```python
from build123d import *

# Parameters (mm, degrees)
F0_R     = 10.3251
F1_DEPTH = 7.9375
F2_W     = 63.5
F2_H     = 7.9375
F3_DEPTH = 68.2625
F4_R     = 9.92251
F5_DEPTH = 88.901
F7_DEPTH = 139.701
F8_DEPTH = 63.5


with BuildPart() as f1:
    # F0 (on Top) → F1 (new body)
    with BuildSketch(Plane.XY):
        with BuildLine():
            Line((63.5, 44.45), (0, 44.45))
            Line((0, 44.45), (0, -44.45))
            Line((0, -44.45), (63.5, -44.45))
            Line((63.5, -44.45), (63.5, -28.575))
            ThreePointArc((63.5, -28.575), (65.359872, -24.084872), (69.85, -22.225))
            Line((69.85, -22.225), (117.475, -22.225))
            ThreePointArc((117.475, -22.225), (139.7, 0), (117.475, 22.225))
            Line((117.475, 22.225), (69.85, 22.225))
            ThreePointArc((69.85, 22.225), (65.359872, 24.084872), (63.5, 28.575))
            Line((63.5, 28.575), (63.5, 44.45))
        make_face()
        with Locations((79.375, 0)):
            Circle(F0_R, mode=Mode.SUBTRACT)
        with Locations((117.475, 0)):
            Circle(F0_R, mode=Mode.SUBTRACT)
    extrude(amount=F1_DEPTH)

    # F2 (on face) → F3 (join)
    with BuildSketch(Plane.XY.offset(7.9375)):
        with Locations((31.75, -40.48125)):
            Rectangle(F2_W, F2_H)
        with Locations((31.75, 40.48125)):
            Rectangle(F2_W, F2_H)
    extrude(amount=F3_DEPTH)

    # F4 (on face) → F5 (cut, through all)
    with BuildSketch(Plane.XZ.offset(44.45)):
        with BuildLine():
            ThreePointArc((0, 44.45), (9.29936, 66.90064), (31.75, 76.2))
            Line((31.75, 76.2), (0, 76.2))
            Line((0, 76.2), (0, 44.45))
        make_face()
        with BuildLine():
            ThreePointArc((31.75, 76.2), (54.20064, 66.90064), (63.5, 44.45))
            Line((63.5, 44.45), (63.5, 76.2))
            Line((63.5, 76.2), (31.75, 76.2))
        make_face()
        with Locations((31.75, 44.45)):
            Circle(F4_R)
    extrude(amount=-F5_DEPTH, mode=Mode.SUBTRACT)

    # F6 (on Right) → F7 (cut, through all)
    with BuildSketch(Plane.YZ):
        with BuildLine():
            ThreePointArc((-31.75, 0), (-40.730256, 3.719744), (-44.45, 12.7))
            Line((-44.45, 12.7), (-44.45, 0))
            Line((-44.45, 0), (-31.75, 0))
        make_face()
        with BuildLine():
            ThreePointArc((44.45, 12.7), (40.730256, 3.719744), (31.75, 0))
            Line((31.75, 0), (44.45, 0))
            Line((44.45, 0), (44.45, 12.7))
        make_face()
    extrude(amount=F7_DEPTH, mode=Mode.SUBTRACT)

    # F6 (on Right) → F8 (join)
    with BuildSketch(Plane.YZ):
        with BuildLine():
            ThreePointArc((36.5125, 12.7), (35.117596, 9.332404), (31.75, 7.9375))
            Line((31.75, 7.9375), (36.5125, 7.9375))
            Line((36.5125, 7.9375), (36.5125, 12.7))
        make_face()
        with BuildLine():
            ThreePointArc((-31.75, 7.9375), (-35.117596, 9.332404), (-36.5125, 12.7))
            Line((-36.5125, 12.7), (-36.5125, 7.9375))
            Line((-36.5125, 7.9375), (-31.75, 7.9375))
        make_face()
    extrude(amount=F8_DEPTH)


solid = f1.part
```
Geometry: final body of the model. Coordinates: model frame, mm. A direction names the side the tool comes from. Round coordinates to 2 decimals unless told otherwise and drop trailing zeros. Loops run counter-clockwise (first coordinate to the right, second up) from the corner with the lowest first, then second, coordinate; pieces in that order, holes last. Notation, with made-up numbers: (82.25, 11.25) -> (97.25, 11.25) arc R13 ccw to (97.25, 26.25) -> close; hole circle Ø5 at (-39.75, 64). An arc over 180 degrees is marked (long way). Use one line per item in the form item = value. Start each with the question number.
1) Section B-B on y = 0. Output: boundary loops of the cut face in (x, z).
2) Access query for faces 4 (the cylindrical face through (127.323, 3.101, 3.913)), 5 (the flat face through (63.5, -38, 22)), 6 (the cylindrical face through (31, -41, 4)), 7 (the cylindrical face through (31.306, -35.08, 9.296)), 8 (the flat face through (94, 22.225, 4)). Directions: +Z, -Z, +X, -X, +Y, -Y. A direction counts if a zero-diameter tool reaches every point of the face in a straight line with its end or side. Return the directions, or none.
3) Section A-A on z = 31.5. Output: boundary loops of the cut face in (x, y), then the cut area to 3 significant figures.
4) First-contact query: P1, Ø6.5, axis at x = 99.5, z = 3, coming from the -Y side (3 decimals); P2, Ø5, axis at y = -37.5, z = 20, coming from the +X side; P3, Ø4, axis at x = 86, z = 5, coming from the +Y side (3 decimals); P4, Ø1, axis at x = 64, y = 1, coming from the -Z side. Flat tips, straight axial feed; report the tip coordinate or a pass-through.
5) Section C-C on z = 41. Output: boundary loops of the cut face in (x, y), then the cut area to 3 significant figures.
6) Draft query along X for faces 1 (the flat face through (53, 0, 7.938)), 2 (the cylindrical face through (36.329, 40.426, 35.647)), 3 (the flat face through (63.5, 38, 23)). Return one class per face: released by +X, released by -X, zero draft, split by the parting line, or undercut.
7) Line query: L1, parallel to Y at x = 21, z = 30.5; L2, parallel to Z at x = 89.5, y = -19.5; L3, parallel to Z at x = 31.75, y = -39.5. Output: solid intervals per line, ascending.
8) Section D-D on z = 10. Output: boundary loops of the cut face in (x, y), then the cut area to 3 significant figures.
Response:
q1.outline = (0, 0) -> (69.05, 0) -> (69.05, 7.94) -> (0, 7.94) -> close; (89.7, 0) -> (107.15, 0) -> (107.15, 7.94) -> (89.7, 7.94) -> close; (127.8, 0) -> (139.7, 0) -> (139.7, 7.94) -> (127.8, 7.94) -> close
q2.face_4 = +Z, -Z
q2.face_5 = +Z, -Z, +X, -Y
q2.face_6 = -Z, +X, -X, -Y
q2.face_7 = +Z, +X, -X
q2.face_8 = +Z, -Z, +X, +Y
q3.outline = (0, -44.45) -> (63.5, -44.45) -> (63.5, -36.51) -> (0, -36.51) -> close; (0, 36.51) -> (63.5, 36.51) -> (63.5, 44.45) -> (0, 44.45) -> close
q3.area = 1,010 mm^2
q4.P1 = -22.225
q4.P2 = 63.5
q4.P3 = 22.225
q4.P4 = 0
q5.outline = (0, -44.45) -> (22.45, -44.45) -> (22.45, -36.51) -> (0, -36.51) -> close; (0, 36.51) -> (22.45, 36.51) -> (22.45, 44.45) -> (0, 44.45) -> close; (41.05, -44.45) -> (63.5, -44.45) -> (63.5, -36.51) -> (41.05, -36.51) -> close; (41.05, 36.51) -> (63.5, 36.51) -> (63.5, 44.45) -> (41.05, 44.45) -> close
q5.area = 713 mm^2
q6.face_1 = zero draft
q6.face_2 = undercut
q6.face_3 = released by +X
q7.L1 = -44.45 to -36.51, 36.51 to 44.45
q7.L2 = 0 to 7.94
q7.L3 = 2.64 to 34.53, 54.37 to 76.2
q8.outline = (0, -44.16) -> (63.5, -44.16) -> (63.5, -35.67) -> (0, -35.67) -> close; (0, 35.67) -> (63.5, 35.67) -> (63.5, 44.16) -> (0, 44.16) -> close
q8.area = 1,080 mm^2
